Check sheet for the modelled part. Datum: model origin and axes. Units: mm. A direction names the side the tool comes from. Round coordinates to 2 decimals unless told otherwise and drop trailing zeros. Order: outer loops, then holes, each group sorted by start corner. A loop starts at its lowest first (then second) coordinate and runs counter-clockwise, first axis right, second up. Notation, with made-up numbers: (55, 58.5) -> (96, 58.5) arc R10 cw to (96, 64.5) -> close; hole circle Ø3 at (37.25, 79). An arc over 180 degrees is marked (long way). Answer as CSV lines item,"result". Start each with the question number.
Autodesk Inventor part; units mm, degrees
ref_plane "YZ Plane" through (0, 0, 0) normal (1, 0, 0) x (0, 1, 0)
ref_plane "XZ Plane" through (0, 0, 0) normal (0, 1, 0) x (-1, 0, 0)
ref_plane "XY Plane" through (0, 0, 0) normal (0, 0, 1) x (1, 0, 0)
sketch "Sketch1" plane through (0, 0, 0) normal (0, 1, 0) x (-1, 0, 0)
  line L0 (0, 0) -> (25.4, 0)
  line L1 (25.4, 0) -> (25.4, 25.4)
  line L2 (25.4, 25.4) -> (0, 25.4)
  line L3 (0, 25.4) -> (0, 0)
  line L4 (3.175, 22.225) -> (22.225, 22.225)
  line L5 (22.225, 22.225) -> (22.225, 3.175)
  line L6 (22.225, 3.175) -> (3.175, 3.175)
  line L7 (3.175, 3.175) -> (3.175, 22.225)
  dimension "d0" = 25.4
  dimension "d1" = 25.4
  dimension "d4" = 3.175
  dimension "d5" = 3.175
  dimension "d6" = 3.175
  dimension "d7" = 3.175
extrude "Extrusion1" add sketch "Sketch1" along normal blind 304.8
sketch "Sketch2" plane through (0, 0, 25.4) normal (1, 0, 0) x (0, 0, -1)
  circle A0 centre (12.7, 292.1) radius 3.175
  line L0 (22.225, 304.8) -> (3.175, 304.8)
  line L1 (0, 0) -> (0, 304.8)
  point P0 (25.4, 0)
  dimension "d10" = 6.35
  dimension "d11" = 12.7
  dimension "d12" = 12.7
extrude "Extrusion2" cut sketch "Sketch2" against normal blind 304.8
sketch "Sketch3" plane through (-25.4, 0, 0) normal (-1, 0, 0) x (0, 0, 1)
  circle A0 centre (12.7, 254) radius 3.175
  line L0 (0, 304.8) -> (25.4, 304.8)
  line L1 (0, 0) -> (0, 304.8)
  dimension "d15" = 6.35
  dimension "d16" = 50.8
  dimension "d17" = 12.7
extrude "Extrusion3" cut sketch "Sketch3" against normal blind 25.4
sketch "Sketch4" plane through (-25.4, 0, 25.4) normal (0, 0, 1) x (1, 0, 0)
  line L0 (11.9432, 247.65) -> (11.9432, 304.8) construction
  line L1 (21.4682, 247.65) -> (21.4682, 304.8)
  line L2 (2.4182, 304.8) -> (2.4182, 247.65)
  arc A0 (2.4182, 247.65) -> (21.4682, 247.65) centre (11.9432, 247.65) ccw
  arc A1 (21.4682, 304.8) -> (2.4182, 304.8) centre (11.9432, 304.8) ccw
  line L3 (0, 0) -> (25.4, 0)
  line L4 (0, 0) -> (0, 304.8)
  line L5 (22.225, 304.8) -> (3.175, 304.8)
  point P0 (11.9432, 276.225)
  dimension "d20" = 57.15
  dimension "d22" = 11.9432
  dimension "d23" = 0
  dimension "d24" = 19.05
extrude "Extrusion4" cut sketch "Sketch4" against normal blind 3.175
equation "\"d5\" = d4"
equation "\"d6\" = d4"
equation "\"d7\" = d4"
properties part number "Substitute Sucker Arm"
1) Access from +Z, -Z, +X, -X, +Y, -Y to the whole of each face (thin tool, end or side, straight path). Record for faces 4 (the face through (-13.666, 238.127, 23.835)), 5 (the face through (-13, 116, 22.225)), 6 (the face through (-1.61, 250.9, 12.01)).
2) Mould release check, pull along Y, two halves, no side actions. Record for faces 1 (the face through (-14, 304.8, 2)), 2 (the face through (-13, 150, 0)), 3 (the face through (-1.57, 295.25, 13.11)): released by +Y, released by -Y, zero draft, split by the parting line, or undercut.
3) Section check A-A on y = 254. Record the cut outline in (x, z) (3 decimals).
4) Material ranges on line 1 along Y through (x, z) = (-2.25, 12.7) (3 decimals); line 2 along Z through (x, y) = (-24.1, 254) (3 decimals); line 3 along X through (y, z) = (201, 7.5) (3 decimals), recorded low to high.
5) Depth check by flat-ended pin: pin 1 Ø5.5 at (y, z) = (254, 12.7) entering from -X; pin 2 Ø0.6 at (x, y) = (-22.5, 289.5) entering from +Z (3 decimals). Enter the tip coordinate at first touch or a pass-through.
6) Section check B-B on z = 12.7. Record the cut outline in (x, y) (3 decimals).
7) Section check C-C on y = 219. Record the cut outline in (x, z) (3 decimals), then the cut area to 3 significant figures.
Solutions:
1,face 4,"+Z, +Y"
1,face 5,"+Y, -Y"
1,face 6,"+X, -X"
2,face 1,"released by +Y"
2,face 2,"zero draft"
2,face 3,"undercut"
3,outline,"(-25.4, 0) -> (0, 0) -> (0, 9.525) -> (-3.175, 9.525) -> (-3.175, 3.175) -> (-22.225, 3.175) -> (-22.225, 9.525) -> (-25.4, 9.525) -> close; (-25.4, 15.875) -> (-22.225, 15.875) -> (-22.225, 22.225) -> (-22.982, 22.225) -> (-22.982, 25.4) -> (-25.4, 25.4) -> close; (-3.932, 22.225) -> (-3.175, 22.225) -> (-3.175, 15.875) -> (0, 15.875) -> (0, 25.4) -> (-3.932, 25.4) -> close"
4,line 1,"y = 0 to 250.825, 257.175 to 288.925, 295.275 to 304.8"
4,line 2,"z = 0 to 9.525, 15.875 to 25.4"
4,line 3,"x = -25.4 to -22.225, -3.175 to 0"
5,pin 1,"passes through"
5,pin 2,"stops at z = 22.225"
6,outline,"(-25.4, 0) -> (-22.225, 0) -> (-22.225, 250.825) -> (-25.4, 250.825) -> close; (-25.4, 257.175) -> (-22.225, 257.175) -> (-22.225, 288.925) -> (-25.4, 288.925) -> close; (-25.4, 295.275) -> (-22.225, 295.275) -> (-22.225, 304.8) -> (-25.4, 304.8) -> close; (-3.175, 0) -> (0, 0) -> (0, 250.825) -> (-3.175, 250.825) -> close; (-3.175, 257.175) -> (0, 257.175) -> (0, 288.925) -> (-3.175, 288.925) -> close; (-3.175, 295.275) -> (0, 295.275) -> (0, 304.8) -> (-3.175, 304.8) -> close"
7,outline,"(-25.4, 0) -> (0, 0) -> (0, 25.4) -> (-25.4, 25.4) -> close; hole (-22.225, 3.175) -> (-3.175, 3.175) -> (-3.175, 22.225) -> (-22.225, 22.225) -> close"
7,area,"282 mm^2"
